Autodesk Inventor part; units mm, degrees
ref_plane "YZ Plane" through (0, 0, 0) normal (1, 0, 0) x (0, 1, 0)
ref_plane "XZ Plane" through (0, 0, 0) normal (0, 1, 0) x (-1, 0, 0)
ref_plane "XY Plane" through (0, 0, 0) normal (0, 0, 1) x (1, 0, 0)
sketch "Esquisse1" plane through (0, 0, 0) normal (0, 1, 0) x (-1, 0, 0)
  line L0 (0, 0) -> (32, 0) construction
  line L1 (32, 0) -> (16, 27.7128) construction
  line L2 (16, 27.7128) -> (0, 0) construction
  line L3 (-10.3913, 17.9982) -> (9.0252, -15.6322) construction
  line L4 (8, -13.8564) -> (32, 0) construction
  line L5 (8, -13.8564) -> (14.9282, -9.8564) construction
  line L6 (8, -13.8564) -> (-10, 17.3205) construction
  line L7 (-10, 17.3205) -> (1.6913, 24.0705) construction
  line L8 (1.6913, 24.0705) -> (4.9413, 18.4413) construction
  line L9 (4.9413, 18.4413) -> (8.9413, 11.5131) construction
  line L10 (8.9413, 11.5131) -> (12.9413, 4.5849) construction
  line L11 (12.9413, 4.5849) -> (16.9413, -2.3433) construction
  circle A0 centre (8.9413, 11.5131) radius 1
  circle A1 centre (12.9413, 4.5849) radius 1
  circle A2 centre (16.9413, -2.3433) radius 1
  circle A3 centre (14.9282, -9.8564) radius 1
  circle A4 centre (4.9413, 18.4413) radius 1
  circle A5 centre (-14.4413, -1.9869) radius 1
  circle A6 centre (-10.4413, -8.9151) radius 1
  circle A7 centre (-6.4413, -15.8433) radius 1
  circle A8 centre (1.0718, -17.8564) radius 1
  circle A9 centre (-18.4413, 4.9413) radius 1
  circle A10 centre (-10, 17.3205) radius 11.6 construction
  line L12 (32, 0) -> (36, -6.9282) construction
  line L13 (36.0415, 0) -> (34.0207, -3.5) construction
  line L14 (34.0207, -3.5) -> (29.9793, -3.5) construction
  line L15 (29.9793, -3.5) -> (27.9585, 0) construction
  line L16 (27.9585, 0) -> (29.9793, 3.5) construction
  line L17 (29.9793, 3.5) -> (34.0207, 3.5) construction
  line L18 (34.0207, 3.5) -> (36.0415, 0) construction
  line L19 (34.0207, 3.5) -> (34.0207, -3.5) construction
  circle A11 centre (16, 27.7128) radius 2
  circle A12 centre (32, 0) radius 2
  line L20 (32, 0) -> (38.9282, 4) construction
  line L21 (-6.4413, -15.8433) -> (-13.3695, -19.8433) construction
  line L22 (42.9282, -2.9282) -> (-6.6195, -31.5346)
  line L23 (-6.6195, -31.5346) -> (-30.6195, 10.0346)
  line L24 (-30.6195, 10.0346) -> (18.9282, 38.641)
  line L25 (18.9282, 38.641) -> (42.9282, -2.9282)
  line L26 (8, -13.8564) -> (12, -20.7846) construction
  line L27 (16, 27.7128) -> (12, 34.641) construction
  circle A13 centre (0, 0) radius 2
  dimension "d0" = 32
  dimension "d1" = 32
  dimension "d2" = 60
  dimension "d4" = 8
  dimension "d6" = 36
  dimension "d7" = 13.5
  dimension "d8" = 6.5
  dimension "d9" = 8
  dimension "d10" = 8
  dimension "d11" = 8
  dimension "d13" = 2
  dimension "d14" = 11.6
  dimension "d15" = 8
  dimension "d16" = 7
  dimension "d17" = 4
  dimension "d19" = 8
  dimension "d20" = 8
  dimension "d26" = 8
  dimension "d27" = 8
extrude "Extrusion1" add sketch "Esquisse1" along normal blind 12
sketch "Esquisse5" plane through (0, 12, 0) normal (0, 1, 0) x (1, 0, 0)
  circle A0 centre (-32, 0) radius 2
  circle A1 centre (-16, -27.7128) radius 2
  line L0 (-42.9282, 2.9282) -> (-18.9282, -38.641)
  line L1 (-27.9585, 0) -> (-29.9793, -3.5)
  line L2 (-29.9793, -3.5) -> (-34.0207, -3.5)
  line L3 (-34.0207, -3.5) -> (-36.0415, 0)
  line L4 (-36.0415, 0) -> (-34.0207, 3.5)
  line L5 (-34.0207, 3.5) -> (-29.9793, 3.5)
  line L6 (-29.9793, 3.5) -> (-27.9585, 0)
  line L7 (-18.0207, -24.2128) -> (-13.9793, -24.2128)
  line L8 (-13.9793, -24.2128) -> (-11.9585, -27.7128)
  line L9 (-11.9585, -27.7128) -> (-13.9793, -31.2128)
  line L10 (-13.9793, -31.2128) -> (-18.0207, -31.2128)
  line L11 (-18.0207, -31.2128) -> (-20.0415, -27.7128)
  line L12 (-20.0415, -27.7128) -> (-18.0207, -24.2128)
  line L13 (-4.0415, 0) -> (-2.0207, 3.5)
  line L14 (-2.0207, 3.5) -> (2.0207, 3.5)
  line L15 (2.0207, 3.5) -> (4.0415, 0)
  line L16 (4.0415, 0) -> (2.0207, -3.5)
  line L17 (2.0207, -3.5) -> (-2.0207, -3.5)
  line L18 (-2.0207, -3.5) -> (-4.0415, 0)
  line L19 (-13.9793, -24.2128) -> (-20.0415, -27.7128) construction
  point P0 (0, 0)
  point P1 (0, 0)
  dimension "d51" = 7
extrude "Extrusion2" cut sketch "Esquisse5" against normal blind 3
sketch "Esquisse6" plane through (0, 12, 0) normal (0, 1, 0) x (1, 0, 0)
  circle A0 centre (18.4413, -4.9413) radius 1
  circle A1 centre (-4.9413, -18.4413) radius 1
  line L0 (-18.9282, -38.641) -> (30.6195, -10.0346)
  line L1 (30.6195, -10.0346) -> (6.6195, 31.5346)
  line L2 (18.4413, -4.9413) -> (21.6913, -10.5705) construction
  line L3 (21.6913, -10.5705) -> (10, -17.3205) construction
  circle A2 centre (10, -17.3205) radius 12 construction
  line L4 (-11.9585, -27.7128) -> (-8.9689, -32.891) construction
  line L5 (-42.9282, 2.9282) -> (-18.9282, -38.641)
  circle A3 centre (-4.9413, -18.4413) radius 2.9833 construction
  line L6 (-8.9689, -32.891) -> (-2.2843, -19.7979)
  arc A4 (-2.2843, -19.7979) -> (-1.9664, -18.2182) centre (-4.9413, -18.4413) ccw
  circle A5 centre (18.4413, -4.9413) radius 2.9833 construction
  line L7 (19.933, -7.525) -> (26.8612, -3.525)
  arc A6 (16.7606, -7.4062) -> (-1.9664, -18.2182) centre (10, -17.3205) ccw
  arc A7 (16.7606, -7.4062) -> (19.933, -7.525) centre (18.4413, -4.9413) ccw
  point P0 (0, 0)
  dimension "d39" = 12
  dimension "d37" = 6.5
  dimension "d38" = 13.5
extrude "Extrusion3" cut sketch "Esquisse6" against normal through all contours L6 A4 A6 A7 L7 L1 L0
fillet "Congé3" radius 10 1 edges at (-8.9689, 6, 32.891)
fillet "Congé4" radius 8 1 edges at (26.8612, 6, 3.525)
fillet "Congé5" radius 8 1 edges at (6.6195, 6, -31.5346)
fillet "Congé6" radius 8 1 edges at (-18.9282, 6, 38.641)
fillet "Congé7" radius 8 1 edges at (-42.9282, 6, -2.9282)
properties part number "joint3+ax12imprint"
Here's how the part is built. I have some questions about the finished solid (model axes, mm). A direction names the side the tool comes from. Round coordinates to 2 decimals unless told otherwise and drop trailing zeros. Order: outer loops, then holes, each group sorted by start corner. A loop starts at its lowest first (then second) coordinate and runs counter-clockwise, first axis right, second up. Notation, with made-up numbers: M 27,16 L 83,16 A14 cw 83,41 Z; hole C -22.75,63 d6. An arc over 180 degrees is marked long. Answer in a Markdown table with one row per item.
Item 1: Imagine slicing it at A-A, the plane x = -32. Write out the boundary of the cut face in (y, z), and give its area (3 significant figures).
A:
| item | result |
|---|---|
| outline | M 0,-9.24 L 12,-9.24 L 12,-3.5 L 9,-3.5 L 9,-2 L 0,-2 Z; M 0,2 L 9,2 L 9,3.5 L 12,3.5 L 12,16 L 0,16 Z |
| area | 246 mm2 |
Item 2: Imagine slicing it at C-C, the plane x = 1. Write out the boundary of the cut face in (y, z).
A:
| item | result |
|---|---|
| outline | M 0,-28.14 L 12,-28.14 L 12,-3.5 L 9,-3.5 L 9,-1.73 L 0,-1.73 Z; M 0,1.73 L 9,1.73 L 9,3.5 L 12,3.5 L 12,9.38 L 0,9.38 Z |
Item 3: Imagine slicing it at D-D, the plane z = 21. Write out the boundary of the cut face in (x, y).
A:
| item | result |
|---|---|
| outline | M -29.11,0 L -2.9,0 L -2.9,12 L -29.11,12 Z |
Item 4: If I drill on L1, parallel to X at y = 10, z = 4.5; L2, parallel to X at y = 10.75, z = 2; L3, parallel to Z at x = -33, y = 9.5, over which ranges is the centre line in solid material (lowest first)? Write a range as from..to.
A:
| item | result |
|---|---|
| L1 | x = -38.64..-13.94, -11.94..17.54, 19.34..22.92 |
| L2 | x = -39.75..-34.89, -29.11..-2.89, 2.89..23.81 |
| L3 | z = -8.66..-3.5, 3.5..14.27 |
Item 5: Thinking about a two-plate mould opening in X: for faces 3 (the face through (-4.99, 6.08, 25.1)), 4 (the face through (-18.155, 6.084, 35.417)), 5 (the face through (-32, 11, -3.5)), which applies, +X half, -X half, draft (parallel to the pull), parting line (faces both ways), or undercut?
A:
| item | result |
|---|---|
| face 3 | +X half |
| face 4 | parting line |
| face 5 | undercut |
Item 6: I'm going to push flat-ended pins straight in: pin 1 (4 mm diameter, centred on x = 8, y = 4, fed in from -Z); pin 2 (3 mm diameter, centred on x = -5.5, y = 2.5, fed in from -Z); pin 3 (6 mm diameter, centred on y = 2, z = -2.5, fed in from -X); pin 4 (1.2 mm diameter, centred on x = -8.94, z = 11.51, fed in from +Y). Where does each tip first touch, or does it pass through?
A:
| item | result |
|---|---|
| pin 1 | stops at z = -28.27 |
| pin 2 | stops at z = -25.4 |
| pin 3 | stops at x = -40 |
| pin 4 | passes through |
Item 7: For faces 1 (the face through (-3, 10.5, 1.8)), 2 (the face through (-9.252, 5.916, 32.567)), which set-ups out of +Z, -Z, +X, -X, +Y, -Y let a thin tool reach every point of the face, with its end or its side?
A:
| item | result |
|---|---|
| face 1 | +Y |
| face 2 | +Z, +X, +Y, -Y |
Item 8: Imagine slicing it at B-B, the plane y = 3.25. State how many separate pieces and enclosed holes the cut face has, and give its area (3 significant figures).
A:
| item | result |
|---|---|
| separate pieces | 1 |
| enclosed holes | 13 |
| area | 2,180 mm2 |
